Here's how the part is built. I have some questions about the finished solid (model axes, mm). Face numbers are marked on the shaded views. A direction names the side the tool comes from. Coordinates: 2 decimals unless noted, no trailing zeros. Order: outer loops, then holes, each group sorted by start corner. A loop starts at its lowest first (then second) coordinate and runs counter-clockwise, first axis right, second up.
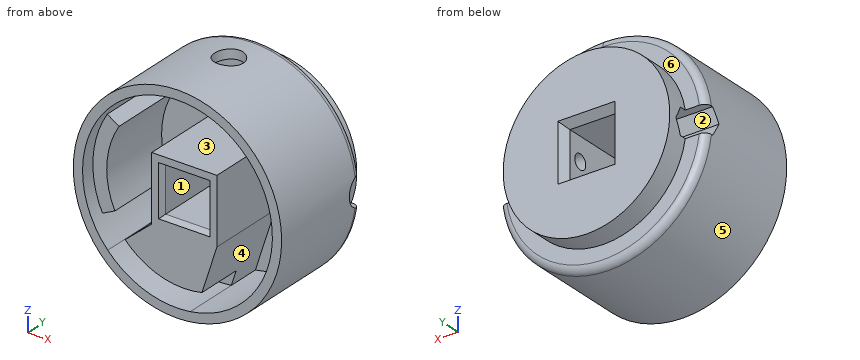
```python
from build123d import *
from OCP.BRepFilletAPI import BRepFilletAPI_MakeChamfer

# Parameters (mm, degrees)
SKETCH1_R                = 22.5
BOSS_EXTRUDE1_DEPTH      = 28
SKETCH2_W                = 10.1
SKETCH2_H                = 10.1
CUT_EXTRUDE2_DEPTH       = 43.385138905
SHELL3_T                 = -2
SKETCH3_R                = 3.1
CUT_EXTRUDE3_DEPTH       = 47.51292831
CHAMFER1_SIZE            = 2
CHAMFER1_SIZE2           = 1.154700538
BOSS_EXTRUDE8_START      = 23
BOSS_EXTRUDE8_DEPTH      = 23
BOSS_EXTRUDE4_DEPTH      = 20
BOSS_EXTRUDE6_DEPTH      = 26
CUT_EXTRUDE5_DEPTH       = 12
CUT_EXTRUDE9_DEPTH       = 2
BOSS_EXTRUDE10_START     = 7
BOSS_EXTRUDE10_DEPTH     = 7
SKETCH21_OUTSIDE_W       = 61.262
SKETCH21_OUTSIDE_H       = 63.965
SKETCH21_OUTSIDE_R       = 18
CUT_EXTRUDE11_DEPTH      = 4.8
CUT_EXTRUDE12_DEPTH      = 47.67125763
CUT_EXTRUDE12_DEPTH_BACK = 47.67125763
SKETCH22_R               = 1.6
CUT_EXTRUDE13_START      = -8.5
SKETCH24_R               = 3.25
CUT_EXTRUDE13_DEPTH      = 39.17125769
CUT_EXTRUDE14_START      = -8.5
CUT_EXTRUDE14_DEPTH      = 39.171257692
FILLET1_R                = 1.5
SKETCH26_R               = 43.919943133
SKETCH26_R_2             = 22.5
CUT_EXTRUDE15_DEPTH      = 44.879993089
CHAMFER2_SIZE            = 0.5
CHAMFER2_SIZE2           = 1.37373871


with BuildPart() as part:
    # Sketch1 → Boss-Extrude1 (new body)
    with BuildSketch(Plane(origin=(0, 0, 0), x_dir=(1, 0, 0), z_dir=(0, 1, 0))):
        with Locations(Location((0, 0, 0), (0, 0, 270))):
            Circle(SKETCH1_R)
    extrude(amount=BOSS_EXTRUDE1_DEPTH)

    # Sketch2 → Cut-Extrude2 (cut, through all)
    with BuildSketch(Plane.XZ):
        Rectangle(SKETCH2_W, SKETCH2_H)
    extrude(amount=-CUT_EXTRUDE2_DEPTH, mode=Mode.SUBTRACT)

    # Shell3
    shell3_openings = [part.faces().sort_by_distance(p)[0] for p in [
        (0, 0, -21.863603897),
    ]]
    offset(amount=SHELL3_T, openings=shell3_openings, kind=Kind.INTERSECTION)

    # Sketch3 → Cut-Extrude3 (cut, through all)
    with BuildSketch(Plane.XY.offset(7.05)):
        with Locations(Location((0, 15, 0), (0, 0, 270.000000016))):
            Circle(SKETCH3_R)
    extrude(amount=CUT_EXTRUDE3_DEPTH, mode=Mode.SUBTRACT)

    # Chamfer1: one chamfer whose edges measure the first distance from different faces: ONE call of the kernel's chamfer builder (chamfer() names one face for all edges)
    chamfer1_edges_1 = [part.edges().sort_by_distance(p)[0] for p in [
        (5.05, 28, 0),
    ]]
    chamfer1_side_1 = [part.faces().sort_by_distance(p)[0] for p in [
        (5.05, 14, 0),
    ]]
    chamfer1_edges_2 = [part.edges().sort_by_distance(p)[0] for p in [
        (0, 28, -5.05),
    ]]
    chamfer1_side_2 = [part.faces().sort_by_distance(p)[0] for p in [
        (0, 14, -5.05),
    ]]
    chamfer1_edges_3 = [part.edges().sort_by_distance(p)[0] for p in [
        (-5.05, 28, 0),
    ]]
    chamfer1_side_3 = [part.faces().sort_by_distance(p)[0] for p in [
        (-5.05, 14, 0),
    ]]
    chamfer1_edges_4 = [part.edges().sort_by_distance(p)[0] for p in [
        (0, 28, 5.05),
    ]]
    chamfer1_side_4 = [part.faces().sort_by_distance(p)[0] for p in [
        (0, 14, 5.05),
    ]]
    chamfer1 = BRepFilletAPI_MakeChamfer(part.part.solid().wrapped)
    for e in chamfer1_edges_1:
        chamfer1.Add(CHAMFER1_SIZE, CHAMFER1_SIZE2, e.wrapped, chamfer1_side_1[0].wrapped)  # the first distance lies on this face
    for e in chamfer1_edges_2:
        chamfer1.Add(CHAMFER1_SIZE, CHAMFER1_SIZE2, e.wrapped, chamfer1_side_2[0].wrapped)  # the first distance lies on this face
    for e in chamfer1_edges_3:
        chamfer1.Add(CHAMFER1_SIZE, CHAMFER1_SIZE2, e.wrapped, chamfer1_side_3[0].wrapped)  # the first distance lies on this face
    for e in chamfer1_edges_4:
        chamfer1.Add(CHAMFER1_SIZE, CHAMFER1_SIZE2, e.wrapped, chamfer1_side_4[0].wrapped)  # the first distance lies on this face
    add(Compound.cast(chamfer1.Shape()), mode=Mode.REPLACE)

    # Sketch18 → Boss-Extrude8 (add)
    with BuildSketch(Plane.XZ.offset(-26).offset(BOSS_EXTRUDE8_START)):
        with BuildLine():
            Line((-15.72889581, -7.671495069), (-18.425277949, -8.986608509))
            ThreePointArc((-18.425277949, -8.986608509), (-20.471905462, 1.072887103), (-17.384985971, 10.863344917))
            Line((-17.384985971, 10.863344917), (-14.840841683, 9.273587124))
            ThreePointArc((-14.840841683, 9.273587124), (-17.476016858, 0.915879234), (-15.72889581, -7.671495069))
        make_face()
    extrude(amount=-BOSS_EXTRUDE8_DEPTH)

    # Sketch9 → Boss-Extrude4 (add)
    with BuildSketch(Plane.XZ):
        Polygon((2.070380013, -22.404542544), (-16.587666088, -15.201951643), (-17.668054723, -18.000658558), (0.989991378, -25.203249459), align=None)
    extrude(amount=-BOSS_EXTRUDE4_DEPTH)

    # Sketch11 → Boss-Extrude6 (add)
    with BuildSketch(Plane.XZ):
        with BuildLine():
            Line((2.070380013, -22.404542544), (7.05, -7.05))
            Line((7.05, -7.05), (-7.05, -7.05))
            Line((-7.05, -7.05), (-16.587666088, -15.201951643))
            ThreePointArc((-16.587666088, -15.201951643), (-8.102914764, -20.990301864), (2.070380013, -22.404542544))
        make_face()
    extrude(amount=-BOSS_EXTRUDE6_DEPTH)

    # Sketch12 → Cut-Extrude5 (cut)
    with BuildSketch(Plane.XZ):
        with BuildLine():
            Line((3.795196001, -17.086112517), (2.74804579, -20.314975863))
            ThreePointArc((2.74804579, -20.314975863), (-6.94389773, -19.288138436), (-15.066327631, -13.901646367))
            Line((-15.066327631, -13.901646367), (-12.785820172, -11.952470714))
            ThreePointArc((-12.785820172, -11.952470714), (-5.176523958, -16.719520129), (3.795196001, -17.086112517))
        make_face()
    extrude(amount=-CUT_EXTRUDE5_DEPTH, mode=Mode.SUBTRACT)

    # Sketch17 → Cut-Extrude9 (cut)
    with BuildSketch(Plane.XZ):
        with BuildLine():
            Line((7.05, 7.05), (7.05, -7.05))
            Line((7.05, -7.05), (3.795196001, -17.086112517))
            ThreePointArc((3.795196001, -17.086112517), (-5.176523958, -16.719520129), (-12.785820172, -11.952470714))
            Line((-12.785820172, -11.952470714), (-7.05, -7.05))
            Line((-7.05, -7.05), (-7.05, 7.05))
            Line((-7.05, 7.05), (7.05, 7.05))
        make_face()
    extrude(amount=-CUT_EXTRUDE9_DEPTH, mode=Mode.SUBTRACT)

    # Sketch20 → Boss-Extrude10 (add)
    with BuildSketch(Plane.XZ.offset(-26).offset(BOSS_EXTRUDE10_START)):
        with BuildLine():
            Line((2.74804579, -20.314975863), (7.05, -7.05))
            Line((7.05, -7.05), (7.05, 7.05))
            Line((7.05, 7.05), (-7.05, 7.05))
            Line((-7.05, 7.05), (-7.05, -7.05))
            Line((-7.05, -7.05), (-15.066327631, -13.901646367))
            ThreePointArc((-15.066327631, -13.901646367), (6.94389773, 19.288138436), (2.74804579, -20.314975863))
        make_face()
    extrude(amount=-BOSS_EXTRUDE10_DEPTH)

    # Sketch21 outside → Cut-Extrude11 (cut)
    with BuildSketch(Plane(origin=(0, 28, 0), x_dir=(1, 0, 0), z_dir=(0, 1, 0))):
        with Locations((0, 1.3515)):
            Rectangle(SKETCH21_OUTSIDE_W, SKETCH21_OUTSIDE_H)
        with Locations(Location((0, 0, 0), (0, 0, 270))):
            Circle(SKETCH21_OUTSIDE_R, mode=Mode.SUBTRACT)
    extrude(amount=-CUT_EXTRUDE11_DEPTH, mode=Mode.SUBTRACT)

    # Sketch22 → Cut-Extrude12 (cut, two sides: drawn at the far end of the back side and taken through both)
    with BuildSketch(Plane.ZY.offset(-5.05).offset(-CUT_EXTRUDE12_DEPTH_BACK)):
        with Locations((0, 23)):
            Circle(SKETCH22_R)
    extrude(amount=CUT_EXTRUDE12_DEPTH + CUT_EXTRUDE12_DEPTH_BACK, mode=Mode.SUBTRACT)

    # Sketch24 → Cut-Extrude13 (cut, through all)
    with BuildSketch(Plane.ZY.offset(-5.05).offset(CUT_EXTRUDE13_START)):
        with Locations((0, 23)):
            Circle(SKETCH24_R)
    extrude(amount=-CUT_EXTRUDE13_DEPTH, mode=Mode.SUBTRACT)

    # Sketch25 → Cut-Extrude14 (cut, through all)
    with BuildSketch(Plane(origin=(-5.05, 0, 0), x_dir=(0, 0, -1), z_dir=(1, 0, 0)).offset(CUT_EXTRUDE14_START)):
        Polygon((0, 19.75), (2.814582562, 21.375), (2.814582562, 24.625), (0, 26.25), (-2.814582562, 24.625), (-2.814582562, 21.375), align=None)
    extrude(amount=-CUT_EXTRUDE14_DEPTH, mode=Mode.SUBTRACT)

    # Fillet1
    # the kernel refuses this fillet: 1.5 mm, written as the material it takes off along each edge
    with BuildSketch(Plane(origin=(0, 23.2, 0), x_dir=(0, 0, 1), z_dir=(1, 0, 0))) as fillet1_piece_1:
        with BuildLine():
            CenterArc((22.5 - FILLET1_R, FILLET1_R), FILLET1_R, 270, 90)
            Line((22.5, FILLET1_R), (22.5, 0))
            Line((22.5, 0), (22.5 - FILLET1_R, 0))
        make_face()
    revolve(axis=Axis((0, 23.2, 0), (0, -1, 0)), revolution_arc=92.366443414, mode=Mode.SUBTRACT)
    with BuildSketch(Plane(origin=(0, 23.2, 0), x_dir=(-0.9991402664664062, 0, 0.041457543649361384), z_dir=(0.041457543649361384, 0, 0.9991402664664062))) as fillet1_piece_2:
        with BuildLine():
            CenterArc((22.5 - FILLET1_R, FILLET1_R), FILLET1_R, 270, 90)
            Line((22.5, FILLET1_R), (22.5, 0))
            Line((22.5, 0), (22.5 - FILLET1_R, 0))
        make_face()
    revolve(axis=Axis((0, 23.2, 0), (0, -1, 0)), revolution_arc=183.648889302, mode=Mode.SUBTRACT)
    with BuildSketch(Plane(origin=(0, 23.2, 0), x_dir=(0.9997569746526436, 0, -0.022045217925738058), z_dir=(-0.022045217925738058, 0, -0.9997569746526436))) as fillet1_piece_3:
        with BuildLine():
            CenterArc((22.5 - FILLET1_R, FILLET1_R), FILLET1_R, 270, 90)
            Line((22.5, FILLET1_R), (22.5, 0))
            Line((22.5, 0), (22.5 - FILLET1_R, 0))
        make_face()
    revolve(axis=Axis((0, 23.2, 0), (0, -1, 0)), revolution_arc=91.263200277, mode=Mode.SUBTRACT)

    # Sketch26 → Cut-Extrude15 (cut, through all)
    with BuildSketch(Plane.XZ):
        Circle(SKETCH26_R)
        with Locations(Location((0, 0, 0), (0, 0, 352.392535773))):
            Circle(SKETCH26_R_2, mode=Mode.SUBTRACT)
    extrude(amount=-CUT_EXTRUDE15_DEPTH, mode=Mode.SUBTRACT)

    # Chamfer2
    chamfer2_edges = [part.edges().sort_by_distance(p)[0] for p in [
        (0, 2, 5.05),
        (-5.05, 2, 0),
        (0, 2, -5.05),
        (5.05, 2, 0),
    ]]
    chamfer2_side = [part.faces().sort_by_distance(p)[0] for p in [
        (-1.341973038, 2, -7.273001119),
    ]]
    chamfer(chamfer2_edges, length=CHAMFER2_SIZE, length2=CHAMFER2_SIZE2, reference=chamfer2_side[0])


solid = part.part
```
Q1. We'd pull the mould along X, two halves only. Please class the marked faces 4, 5 and 6: pulls with the +X half, pulls with the -X half, needs draft (parallel to the pull), parting line crosses it, or undercut.
Q2. If we section it at A-A on y = 5: Write out the boundary of the cut face in (x, z).
Q3. I need wall thicknesses on L1, parallel to Z at x = 0, y = 7; L2, parallel to X at y = 5, z = 0; L3, parallel to Z at x = -3, y = 17. Which ranges of each line are inside material? Lowest first, please.
Q4. Will these pins go through, and if not, where does the flat tip stop? pin 1 (4 mm diameter, centred on y = 7.5, z = 11.5, fed in from -X); pin 2 (3 mm diameter, centred on x = 5.5, z = -1, fed in from -Y); pin 3 (5 mm diameter, centred on y = 5, z = 16, fed in from -X).
Q5. For the marked faces 1, 2 and 3, which set-ups out of +Z, -Z, +X, -X, +Y, -Y let a thin tool reach every point of the face, with its end or its side?
Q6. If we section it at B-B on y = 15: Write out the boundary of the cut face in (x, z).
Reply:
1. face 4: undercut
1. face 5: parting line crosses it
1. face 6: needs draft
2. outline: circle Ø45 at (0, 0); (-12.79, -11.95) arc R17.5 ccw to (3.8, -17.09) - (7.05, -7.05) - (7.05, 7.05) - (-7.05, 7.05) - (-7.05, -7.05) - close; hole (-18.43, -8.99) arc R20.5 ccw (long way) to (-17.38, 10.86) - (-14.84, 9.27) arc R17.5 ccw to (-15.73, -7.67) - close; hole (-5.05, -5.05) - (5.05, -5.05) - (5.05, 5.05) - (-5.05, 5.05) - close
3. L1: z = -22.5 to -20.5, -17.5 to -5.05, 5.05 to 7.05, 20.5 to 22.5
3. L2: x = -22.5 to -17.5, -7.05 to -5.05, 5.05 to 7.05, 20.5 to 22.5
3. L3: z = -22.3 to -5.05, 5.05 to 7.05, 20.28 to 22.3
4. pin 1: stops at x = -20.4
4. pin 2: stops at y = 2
4. pin 3: stops at x = -18
5. face 1: +Y, -Y
5. face 2: -X
5. face 3: -Y
6. outline: (-18.43, -8.99) - (-15.73, -7.67) arc R17.5 cw to (-14.84, 9.27) - (-17.38, 10.86) arc R20.5 cw to (-3.1, 20.26) - (-3.1, 22.29) arc R22.5 ccw (long way) to (3.1, 22.29) - (3.1, 20.26) arc R20.5 cw to (2.75, -20.31) - (7.05, -7.05) - (7.05, 7.05) - (-7.05, 7.05) - (-7.05, -7.05) - (-15.07, -13.9) arc R20.5 cw to start; hole (-5.05, -5.05) - (5.05, -5.05) - (5.05, 5.05) - (-5.05, 5.05) - close
